```python
from build123d import *

# Parameters (mm, degrees)
CROQUIS1_R              = 33
SALIENTE_EXTRUIR1_DEPTH = 16
CROQUIS2_R              = 21
SALIENTE_EXTRUIR2_DEPTH = 7
CROQUIS3_R              = 17
SALIENTE_EXTRUIR3_DEPTH = 1.5
CROQUIS4_R              = 13
CORTAR_EXTRUIR1_DEPTH   = 53.709107372
CHAFL_N1_SIZE           = 1
CROQUIS5_R              = 5.25
CORTAR_EXTRUIR2_DEPTH   = 6.5
CROQUIS6_R              = 3.25
CORTAR_EXTRUIR3_DEPTH   = 49.582404222
MATRIZC1_COUNT          = 4
CHAFL_N2_SIZE           = 1


with BuildPart() as part:
    # Croquis1 → Saliente-Extruir1 (new body)
    with BuildSketch(Plane(origin=(0, 0, 0), x_dir=(1, 0, 0), z_dir=(0, 1, 0))):
        with Locations(Location((0, 0, 0), (0, 0, 270))):
            Circle(CROQUIS1_R)
    extrude(amount=SALIENTE_EXTRUIR1_DEPTH)

    # Croquis2 → Saliente-Extruir2 (add)
    with BuildSketch(Plane(origin=(0, 16, 0), x_dir=(1, 0, 0), z_dir=(0, 1, 0))):
        with Locations(Location((0, 0, 0), (0, 0, 270))):
            Circle(CROQUIS2_R)
    extrude(amount=SALIENTE_EXTRUIR2_DEPTH)

    # Croquis3 → Saliente-Extruir3 (add)
    with BuildSketch(Plane.XZ):
        with Locations(Location((0, 0, 0), (0, 0, 90))):
            Circle(CROQUIS3_R)
    extrude(amount=SALIENTE_EXTRUIR3_DEPTH)

    # Croquis4 → Cortar-Extruir1 (cut, through all)
    with BuildSketch(Plane(origin=(0, 23, 0), x_dir=(1, 0, 0), z_dir=(0, 1, 0))):
        with Locations(Location((0, 0, 0), (0, 0, 270))):
            Circle(CROQUIS4_R)
    extrude(amount=-CORTAR_EXTRUIR1_DEPTH, mode=Mode.SUBTRACT)

    # Chaflán1
    chafl_n1_edges = [part.edges().sort_by_distance(p)[0] for p in [
        (0, 16, -33),
    ]]
    chamfer(chafl_n1_edges, length=CHAFL_N1_SIZE)

    # Croquis5 → Cortar-Extruir2 (cut)
    with BuildSketch(Plane(origin=(0, 16, 0), x_dir=(1, 0, 0), z_dir=(0, 1, 0))):
        with Locations(Location((26.5, 0, 0), (0, 0, 270))):
            Circle(CROQUIS5_R)
    cortar_extruir2 = extrude(amount=-CORTAR_EXTRUIR2_DEPTH, mode=Mode.SUBTRACT)

    # Croquis6 → Cortar-Extruir3 (cut, through all)
    with BuildSketch(Plane(origin=(0, 9.5, 0), x_dir=(1, 0, 0), z_dir=(0, 1, 0))):
        with Locations(Location((26.5, 0, 0), (0, 0, 270))):
            Circle(CROQUIS6_R)
    cortar_extruir3 = extrude(amount=-CORTAR_EXTRUIR3_DEPTH, mode=Mode.SUBTRACT)

    # MatrizC1: Cortar-Extruir2, Cortar-Extruir3 ×4 about axis
    matrizc1_axis = Axis((0, 0, 0), (0, 1, 0))
    add([cortar_extruir2.rotate(matrizc1_axis, i * 360 / MATRIZC1_COUNT) for i in range(1, MATRIZC1_COUNT)], mode=Mode.SUBTRACT)
    add([cortar_extruir3.rotate(matrizc1_axis, i * 360 / MATRIZC1_COUNT) for i in range(1, MATRIZC1_COUNT)], mode=Mode.SUBTRACT)

    # Chaflán2
    chafl_n2_edges = [part.edges().sort_by_distance(p)[0] for p in [
        (0, 23, -21),
    ]]
    chamfer(chafl_n2_edges, length=CHAFL_N2_SIZE)


solid = part.part
```
Source: CAD feature listing. Evaluate the final solid. Frame: model axes, mm. A direction names the side the tool comes from. Round coordinates to 2 decimals unless told otherwise and drop trailing zeros. Write each loop counter-clockwise with the first axis right and the second up, starting at its lowest first coordinate (ties: lowest second). Pieces come first, ordered by that corner, then holes. Notation, with made-up numbers: M 60,-33.5 L 80,-33.5 A18 ccw 80,-4.5 Z; hole C 60,-15 d8. An arc over 180 degrees is marked long. Answer as a JSON object with one key per item and string values. Group by question number.
(1) Ray query, line 1 (X direction, y = 6, z = 0); line 2 (Z direction, x = 0.5, y = 13.5); line 3 (X direction, y = 14, z = 12). Return the intervals inside material, ascending. Write a range as [from, to].
(2) Section query C-C on y = 4.25. Output: boundary loops of the cut face in (x, z), then the cut area to 3 significant figures.
(3) Mould query, pull axis X, two halves, no side actions, for faces 4 (the cylindrical face through (23.327, 4.816, -0.705)), 5 (the cylindrical face through (-0.705, 4.816, -23.327)), 6 (the cylindrical face through (-32.215, 7.395, -7.154)), 7 (the flat face through (-21, 16, 7)). Classes: +X half, -X half, draft (parallel to the pull), parting line (faces both ways), or undercut.
(4) First-contact query: pin 1 (10 mm diameter, centred on y = 12, z = -18, fed in from -X); pin 2 (4 mm diameter, centred on x = 22.5, y = 11.5, fed in from +Z); pin 3 (13.5 mm diameter, centred on x = 26.5, z = 0, fed in from -Y). Flat tips, straight axial feed; report the tip coordinate or a pass-through.
(5) Section query A-A on z = 0. State how many separate pieces and enclosed holes the cut face has, then the cut area to 3 significant figures.
(6) Reachability of faces 1 (the cylindrical face through (-23.327, 4.816, 0.705)), 2 (the flat face through (-14, 0, 14)), 3 (the cylindrical face through (-21.84, 12.8, -2.42)) from +Z, -Z, +X, -X, +Y, -Y: full face, straight path, thin tool, end or side. Return the list, or none.
Computed values:
{
 "1": {"line 1": "[-33, -29.75], [-23.25, -13], [13, 23.25], [29.75, 33]", "line 2": "[-33, -31.73], [-21.27, -12.99], [12.99, 21.27], [31.73, 33]", "line 3": "[-30.74, -5], [5, 30.74]"},
 "2": {"outline": "C 0,0 d66; hole C -26.5,0 d6.5; hole C 0,0 d26; hole C 0,-26.5 d6.5; hole C 0,26.5 d6.5; hole C 26.5,0 d6.5", "area": "2,760 mm^2"},
 "3": {"face 4": "undercut", "face 5": "undercut", "face 6": "parting line", "face 7": "draft"},
 "4": {"pin 1": "x = -30.33", "pin 2": "z = 25.86", "pin 3": "y = 0"},
 "5": {"separate pieces": "4", "enclosed holes": "0", "area": "502 mm^2"},
 "6": {"face 1": "+Y, -Y", "face 2": "-Y", "face 3": "+Y"}
}
